```python
from build123d import *

# Parameters (mm, degrees)
SKETCH2_R             = 1.5
BOSS_EXTRUDE3_DEPTH   = 2
BOSS_EXTRUDE3_2_DEPTH = 2
BOSS_EXTRUDE3_3_DEPTH = 2
BOSS_EXTRUDE3_4_DEPTH = 2
BOSS_EXTRUDE7_DEPTH   = 14.5
BOSS_EXTRUDE8_DEPTH   = 2
BOSS_EXTRUDE9_DEPTH   = 20.5


with BuildPart() as part:
    # Sketch2 → Boss-Extrude3 (new body)
    with BuildSketch(Plane(origin=(0, 0, 0), x_dir=(1, 0, 0), z_dir=(0, 1, 0))):
        with BuildLine():
            Line((-43.230453913, 45.247658967), (-32.051235735, 38.062807212))
            add(Edge.make_bspline(
                [(-32.051235735, 38.062807212), (-29.653859452, 36.522020287), (-32.359204514, 33.058015897), (-34.393292894, 29.162596744), (-36.78390878, 30.699038781)],
                knots=[0, 0, 0, 0, 0.5, 1, 1, 1, 1], degree=3))
            Line((-36.78390878, 30.699038781), (-47.586935967, 37.642113656))
            Line((-47.586935967, 37.642113656), (-43.230453913, 45.247658967))
        make_face()
        with Locations(Location((-36.090252253, 36.336715974, 0), (0, 0, 270))):
            Circle(SKETCH2_R, mode=Mode.SUBTRACT)
    extrude(amount=BOSS_EXTRUDE3_DEPTH)



with BuildPart() as body_2:
    # Sketch2 → Boss-Extrude3 2 (new body)
    with BuildSketch(Plane(origin=(0, 0, 0), x_dir=(1, 0, 0), z_dir=(0, 1, 0))):
        with BuildLine():
            Line((-36.185423109, -25.10610692), (-21.279130416, -14.871322122))
            add(Edge.make_bspline(
                [(-25.795747584, -8.293165489), (-24.143697719, -7.158854283), (-21.111071083, -9.916279371), (-19.518538576, -13.662485091), (-21.279130416, -14.871322122)],
                knots=[0, 0, 0, 0, 0.5, 1, 1, 1, 1], degree=3))
            Line((-25.795747584, -8.293165489), (-40.164732197, -18.159030081))
            Line((-40.164732197, -18.159030081), (-36.185423109, -25.10610692))
        make_face()
        with Locations(Location((-26.079416612, -12.817810533, 0), (0, 0, 270))):
            Circle(SKETCH2_R, mode=Mode.SUBTRACT)
    extrude(amount=BOSS_EXTRUDE3_2_DEPTH)


with BuildPart() as body_3:
    # Sketch2 → Boss-Extrude3 3 (new body)
    with BuildSketch(Plane(origin=(0, 0, 0), x_dir=(1, 0, 0), z_dir=(0, 1, 0))):
        with BuildLine():
            Line((29.211666773, -22.314450198), (14.869230537, -14.260003913))
            ThreePointArc((14.869230537, -14.260003913), (14.264243858, -13.347032924), (14.652672015, -12.322997536))
            Line((14.652672015, -12.322997536), (19.160499642, -8.253264805))
            ThreePointArc((19.160499642, -8.253264805), (19.831311373, -7.951400174), (20.552224713, -8.097669073))
            Line((20.552224713, -8.097669073), (33.205147834, -15.203316117))
            Line((33.205147834, -15.203316117), (29.211666773, -22.314450198))
        make_face()
        with Locations(Location((19.995405598, -13.234640771, 0), (0, 0, 270))):
            Circle(SKETCH2_R, mode=Mode.SUBTRACT)
    extrude(amount=BOSS_EXTRUDE3_3_DEPTH)


with BuildPart() as body_4:
    # Sketch2 → Boss-Extrude3 4 (new body)
    with BuildSketch(Plane(origin=(0, 0, 0), x_dir=(1, 0, 0), z_dir=(0, 1, 0))):
        with BuildLine():
            Line((35.956282792, 42.745174925), (24.662993698, 33.699023938))
            ThreePointArc((24.662993698, 33.699023938), (23.78100089, 33.442857668), (22.976200889, 33.885383856))
            Line((22.976200889, 33.885383856), (19.347327143, 38.415699606))
            ThreePointArc((19.347327143, 38.415699606), (19.091160873, 39.297692414), (19.533687061, 40.102492416))
            Line((19.533687061, 40.102492416), (31.884499443, 49.995740759))
            Line((31.884499443, 49.995740759), (35.956282792, 42.745174925))
        make_face()
        with Locations(Location((24.166347117, 37.603010106, 0), (0, 0, 270))):
            Circle(SKETCH2_R, mode=Mode.SUBTRACT)
    extrude(amount=BOSS_EXTRUDE3_4_DEPTH)


with BuildPart() as part_1:
    add(part.part)

    add(body_2.part)  # Boss-Extrude7 merges body 2

    add(body_3.part)  # Boss-Extrude7 merges body 3

    add(body_4.part)  # Boss-Extrude7 merges body 4
    # Sketch7 → Boss-Extrude7 (add)
    with BuildSketch(Plane.XZ):
        Polygon((-36.185423109, 25.10610692), (-37.920880681, 26.100182881), (-41.900189769, 19.153106042), (-40.164732197, 18.159030081), align=None)
        Polygon((-43.230453913, -45.247658967), (-47.586935967, -37.642113656), (-49.322393538, -38.636189617), (-44.965911485, -46.241734929), align=None)
        Polygon((31.884499443, -49.995740759), (35.956282792, -42.745174925), (37.700117882, -43.724480381), (33.628334533, -50.975046216), align=None)
        Polygon((29.211666773, 22.314450198), (33.205147834, 15.203316117), (34.948982925, 16.182621573), (30.955501863, 23.293755654), align=None)
    extrude(amount=-BOSS_EXTRUDE7_DEPTH)

    # Sketch8 → Boss-Extrude8 (add)
    with BuildSketch(Plane(origin=(0, 14.5, 0), x_dir=(1, 0, 0), z_dir=(0, 1, 0))):
        with BuildLine():
            Line((-83.939033809, -12.743691802), (-67.948382544, -35.953321652))
            Line((-67.948382544, -35.953321652), (-31.333133825, -35.953321652))
            Line((-31.333133825, -35.953321652), (-1.800901789, -33.787598607))
            Line((-1.800901789, -33.787598607), (1.845003483, -35.953321652))
            Line((1.845003483, -35.953321652), (54.392894937, -31.485495915))
            Line((54.392894937, -31.485495915), (59.409090539, -23.040937859))
            Line((59.409090539, -23.040937859), (58.585665433, -5.537982821))
            Line((58.585665433, -5.537982821), (63.277626353, 16.220382558))
            Line((63.277626353, 16.220382558), (58.585665433, 37.978747936))
            Line((58.585665433, 37.978747936), (59.409090539, 55.481702974))
            Line((59.409090539, 55.481702974), (54.392894937, 63.926261031))
            Line((54.392894937, 63.926261031), (1.845003483, 68.394086768))
            Line((1.845003483, 68.394086768), (-1.800901789, 66.228363722))
            Line((-1.800901789, 66.228363722), (-31.333133825, 68.394086768))
            Line((-31.333133825, 68.394086768), (-67.948382544, 68.394086768))
            Line((-67.948382544, 68.394086768), (-83.939033809, 45.184456918))
            Line((-83.939033809, 45.184456918), (-82.229044773, 35.927906641))
            add(Edge.make_bspline(
                [(-82.229044773, 35.927906641), (-81.079922832, 29.707454467), (-80.671423408, 23.540442654), (-80.671423408, 17.253629197)],
                knots=[0, 0, 0, 0, 1, 1, 1, 1], degree=3))
            Line((-80.671423408, 17.253629197), (-80.671423408, 15.187135918))
            add(Edge.make_bspline(
                [(-82.229044773, -3.487141526), (-81.079922832, 2.733310648), (-80.671423408, 8.900322461), (-80.671423408, 15.187135918)],
                knots=[0, 0, 0, 0, 1, 1, 1, 1], degree=3))
            Line((-82.229044773, -3.487141526), (-83.939033809, -12.743691802))
        make_face()
        Polygon((-59.857375923, 16.220382558), (-40.164732197, -18.159030081), (-32.644643784, -31.287598607), (23.993388186, -31.287598607), (50.833438729, 16.220382558), (23.99393098, 63.976016309), (-32.502787546, 63.976016309), align=None, mode=Mode.SUBTRACT)
    extrude(amount=BOSS_EXTRUDE8_DEPTH)

    # Sketch9 → Boss-Extrude9 (add)
    with BuildSketch(Plane.XZ.offset(-14.5)):
        Polygon((-67.948382544, -66.394086768), (-69.326315011, -66.394086768), (-67.948382544, -68.394086768), (-31.333133825, -68.394086768), (-1.800901789, -66.228363722), (1.845003483, -68.394086768), (54.392894937, -63.926261031), (55.648633387, -61.81227723), (54.223458503, -61.933451132), (2.314827743, -66.346924443), (-1.320082635, -64.187732531), (-31.406369708, -66.394086768), align=None)
        Polygon((-67.948382544, 33.953321652), (-69.326315011, 33.953321652), (-67.948382544, 35.953321652), (-31.333133825, 35.953321652), (-1.800901789, 33.787598607), (1.845003483, 35.953321652), (54.392894937, 31.485495915), (55.648633387, 29.371512115), (54.223458503, 29.492686016), (2.314827743, 33.906159327), (-1.320082635, 31.746967416), (-31.406369708, 33.953321652), align=None)
    extrude(amount=BOSS_EXTRUDE9_DEPTH)


solid = part_1.part
```
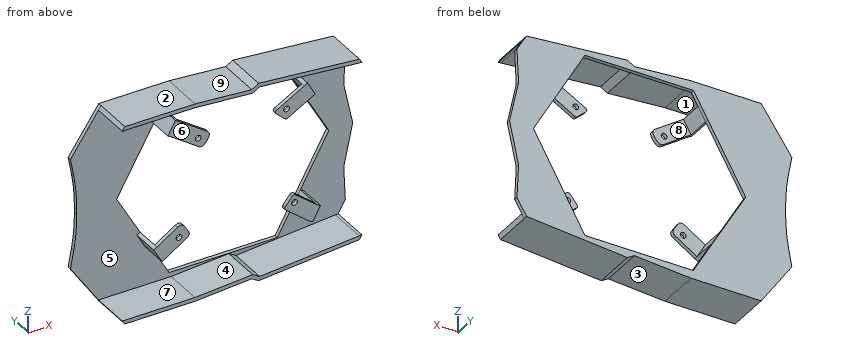
Input: part model. Units: mm. Frame: model coordinates. Face numbers are marked on the shaded views. A direction names the side the tool comes from. Round coordinates to 2 decimals unless told otherwise and drop trailing zeros. Loops run counter-clockwise (first coordinate to the right, second up) from the corner with the lowest first, then second, coordinate; pieces in that order, holes last. Notation, with made-up numbers: (63.25, 71) - (81.25, 71) arc R17 cw to (81.25, 94) - close; hole circle Ø7 at (36.5, 69). An arc over 180 degrees is marked (long way). One line per item, written item: value. Start each with the question number.
(1) Access query for the marked faces 5, 6, 7, 8 and 9. Directions: +Z, -Z, +X, -X, +Y, -Y. A direction counts if a zero-diameter tool reaches every point of the face in a straight line with its end or side. Return the directions, or none.
(2) Section A-A, the plane y = -3.75. Return loops of the section in (x, z) (1 decimal).
(3) Draft query along Z for the marked faces 1, 2, 3 and 4. Return one class per face: +Z half, -Z half, draft (parallel to the pull), parting line (faces both ways), or undercut.
(4) Section D-D, the plane y = 6.5. Count the separate pieces of the cut face and the enclosed holes in it, plus the area to 3 significant figures.
(5) Ray query, line 1 (Z direction, x = -53.5, y = 9.5); line 2 (Z direction, x = -45, y = 1.5); line 3 (Z direction, x = -24, y = 0.25). Return the intervals inside material, ascending. Write a range as [from, to].
(6) Section C-C, the plane x = 6. Return loops of the section in (y, z).
(7) Contact query for flat-ended pins moving along their axis: P1, Ø19.5, axis at x = 25.5, z = -42.5, coming from the -Y side; P2, Ø2, axis at y = 15.5, z = -16.5, coming from the -X side; P3, Ø12, axis at x = -35.5, z = -39, coming from the +Y side; P4, Ø2.5, axis at x = -36.09, z = -36.34, coming from the -Y side. Output: stop coordinate, or through.
(8) Section B-B, the plane x = -12. Return loops of the section in (y, z).
Results below:
1. face 5: -Y
1. face 6: +X, -X, -Y
1. face 7: -X, -Y
1. face 8: +Y
1. face 9: +Z, +Y, -Y
2. outline: (-69.3, -66.4) - (-67.9, -68.4) - (-31.3, -68.4) - (-1.8, -66.2) - (1.8, -68.4) - (54.4, -63.9) - (55.6, -61.8) - (2.3, -66.3) - (-1.3, -64.2) - (-31.4, -66.4) - close; (-69.3, 34) - (-31.4, 34) - (-1.3, 31.7) - (2.3, 33.9) - (55.6, 29.4) - (54.4, 31.5) - (1.8, 36) - (-1.8, 33.8) - (-31.3, 36) - (-67.9, 36) - close
3. face 1: undercut
3. face 2: +Z half
3. face 3: -Z half
3. face 4: undercut
4. separate pieces: 6
4. enclosed holes: 0
4. area: 565 mm^2
5. line 1: [-68.39, -66.39], [33.95, 35.95]
5. line 2: [-68.39, -66.39], [-46.18, -35.98], [33.95, 35.95]
5. line 3: [-67.86, -65.85], [7.96, 16.74], [33.41, 35.42]
6. outline: (-6, -68.04) - (16.5, -68.04) - (16.5, -63.98) - (14.5, -63.98) - (14.5, -66.03) - (-6, -66.03) - close; (-6, 33.59) - (14.5, 33.59) - (14.5, 31.29) - (16.5, 31.29) - (16.5, 35.6) - (-6, 35.6) - close
7. P1: y = 0
7. P2: x = -80.67
7. P3: y = 2
7. P4: through
8. outline: (-6, -66.98) - (16.5, -66.98) - (16.5, -63.98) - (14.5, -63.98) - (14.5, -64.97) - (-6, -64.97) - close; (-6, 32.53) - (14.5, 32.53) - (14.5, 31.29) - (16.5, 31.29) - (16.5, 34.54) - (-6, 34.54) - close
